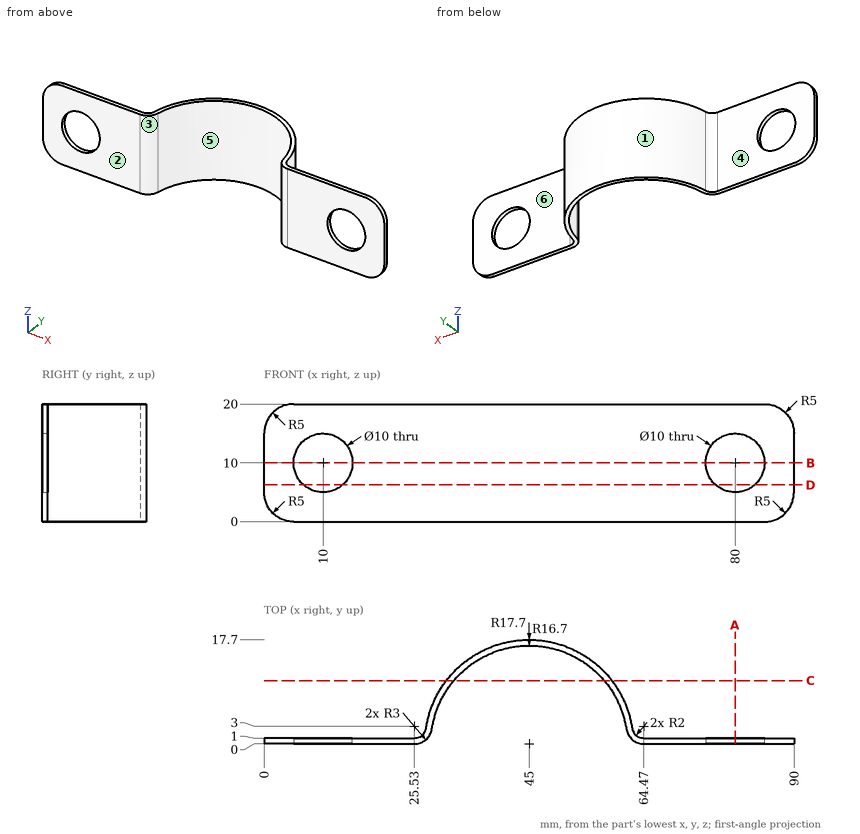
Study the drawing (mm; zero at the part's minimum x, y, z) and answer. A direction names the side the tool comes from. Coordinates: 2 decimals unless noted, no trailing zeros. Write each loop counter-clockwise with the first axis right and the second up, starting at its lowest first coordinate (ties: lowest second). Pieces come first, ordered by that corner, then holes. Notation, with made-up numbers: (-18, 3) -> (5, 3) arc R31 cw to (5, 33) -> close; hole circle Ø7 at (42.25, -5.5). An arc over 180 degrees is marked (long way). Write each question's results on one line, items separated by ' | '. Start each with the question number.
1) A cutting plane is placed at C-C (y = 10.75). Determine the outline of the cut face in (x, z).
2) Flat-ended cylindrical pins translate along their axes: pin 1 Ø10 at (x, z) = (73.5, 16) entering from -Y; pin 2 Ø10 at (x, z) = (37.5, 16) entering from -Y (1 decimal); pin 3 Ø6 at (x, z) = (15.5, 9) entering from +Y; pin 4 Ø1 at (y, z) = (7.5, 13.5) entering from +X. Find the tip coordinate at first contact, or state that the pin passes through.
3) For a pull along X with two mould halves and no side action, classify the marked faces 1, 2 and 3 as +X half, -X half, draft (parallel to the pull), parting line (faces both ways), or undercut.
4) A tool of negligible diameter and unlimited length cuts with its end or side. For the marked faces 4, 5 and 6, from which of +Z, -Z, +X, -X, +Y, -Y can it reach the whole face along a straight path? Write none if from no direction.
5) A cutting plane is placed at A-A (x = 80). Determine the outline of the cut face in (y, z), then the cut area to 3 significant figures.
6) A cutting plane is placed at B-B (z = 10). Determine the outline of the cut face in (x, y) (1 decimal).
7) A cutting plane is placed at D-D (z = 6.25). Determine the outline of the cut face in (x, y) (1 decimal).
8) Straight lines are drawn through the part: probe 1 along Z at (x, y) = (10, 0.7); probe 2 along Y at (x, z) = (19.5, 1.75); probe 3 along X at (y, z) = (14, 19) (1 decimal). For each, find the intervals that lie inside material, in ascending order.
Values follow:
1) outline: (30.94, 0) -> (32.22, 0) -> (32.22, 20) -> (30.94, 20) -> close; (57.78, 0) -> (59.06, 0) -> (59.06, 20) -> (57.78, 20) -> close
2) pin 1: y = 0 | pin 2: y = 11.1 | pin 3: y = 1 | pin 4: x = 61.26
3) face 1: parting line | face 2: draft | face 3: undercut
4) face 4: +Z, -Z, -X, +Y | face 5: +Z, -Z, -Y | face 6: +Z, -Z, +X, +Y
5) outline: (0, 0) -> (1, 0) -> (1, 5) -> (0, 5) -> close; (0, 15) -> (1, 15) -> (1, 20) -> (0, 20) -> close | area: 10.0 mm²
6) outline: (0, 0) -> (5, 0) -> (5, 1) -> (0, 1) -> close; (15, 0) -> (25.5, 0) arc R3 ccw to (28.5, 2.5) arc R16.7 cw to (61.5, 2.5) arc R3 ccw to (64.5, 0) -> (75, 0) -> (75, 1) -> (64.5, 1) arc R2 cw to (62.5, 2.7) arc R17.7 ccw to (27.5, 2.7) arc R2 cw to (25.5, 1) -> (15, 1) -> close; (85, 0) -> (90, 0) -> (90, 1) -> (85, 1) -> close
7) outline: (0, 0) -> (6.7, 0) -> (6.7, 1) -> (0, 1) -> close; (13.3, 0) -> (25.5, 0) arc R3 ccw to (28.5, 2.5) arc R16.7 cw to (61.5, 2.5) arc R3 ccw to (64.5, 0) -> (76.7, 0) -> (76.7, 1) -> (64.5, 1) arc R2 cw to (62.5, 2.7) arc R17.7 ccw to (27.5, 2.7) arc R2 cw to (25.5, 1) -> (13.3, 1) -> close; (83.3, 0) -> (90, 0) -> (90, 1) -> (83.3, 1) -> close
8) probe 1: 0 to 5, 15 to 20 | probe 2: 0 to 1 | probe 3: 34.2 to 35.9, 54.1 to 55.8
